from build123d import *

# Parameters (mm, degrees)
PAD006_DEPTH = 4.5
PAD007_DEPTH = 7


with BuildPart() as part:
    # Sketch015 → Revolution (revolve)
    with BuildSketch(Plane.YZ):
        Polygon((0, 4), (8, 4), (8, 0), (6, 0), (6, -6), (8, -6), (8, -12.5), (11.15, -12.5), (11.15, -39), (3.5, -39), (3.5, -62), (4.5, -62), (4.5, -65), (1.9004150762, -65), (0.5, -67), (0, -67), align=None)
    revolve(axis=Axis((0, 0, 0), (0, 0, 1)))

    # Sketch016 → Pad006 (new body)
    with BuildSketch(Plane.XZ):
        Polygon((-3.5, -62), (-15.5, -62), (-15.5, -42), (4.5, -42), (4.5, -62), (3.5, -62), align=None)
    extrude(amount=PAD006_DEPTH)

    # Sketch016 → Pad007 (join)
    with BuildSketch(Plane.XZ):
        Polygon((-3.5, -62), (-15.5, -62), (-15.5, -42), (4.5, -42), (4.5, -62), (3.5, -62), align=None)
    extrude(amount=-PAD007_DEPTH)


solid = part.part
Work out the finished part from the listing and answer in its coordinate system (mm). A direction names the side the tool comes from. Round coordinates to 2 decimals unless told otherwise and drop trailing zeros. Loops run counter-clockwise (first coordinate to the right, second up) from the corner with the lowest first, then second, coordinate; pieces in that order, holes last. Notation, with made-up numbers: (55, 14.25) - (68, 14.25) arc R11 ccw to (68, 22.25) - close; hole circle Ø1 at (-5.75, -34). An arc over 180 degrees is marked (long way). Use one line per item in the form item = value. Start each with the question number.
(1) Flat-ended cylindrical pins translate along their axes: P1, Ø8, axis at x = -12.5, y = -6.5, coming from the -Z side; P2, Ø6, axis at y = 6.5, z = -39.5, coming from the +X side; P3, Ø10, axis at x = -7.5, z = -57, coming from the +Y side; P4, Ø1, axis at y = -6.5, z = -44, coming from the +X side. Find the tip coordinate at first contact, or state that the pin passes through.
(2) Find section B-B on z = -16. Determine the outline of the cut face in (x, y).
(3) Find section C-C on z = -50. Determine the outline of the cut face in (x, y), and give its area (3 significant figures).
(4) Which of the six approach directions +Z, -Z, +X, -X, +Y, -Y give full straight-line access (tool end or side, diameter ignored) to faces 1 (the face through (-8, 3, -12.5)), 2 (the face through (4, -4, -62)), 3 (the face through (-6, -2, 0))?
(5) Consider line 1 (Z direction, x = -9, y = -2); line 2 (Z direction, x = 1, y = -4); line 3 (Z direction, x = 3.5, y = -8). Determine where each line is inside the solid, lowest interval first.
(6) Find section A-A on z = -40.5. Determine the outline of the cut face in (x, y).
Answer list:
q1.P1 = -62
q1.P2 = 10.57
q1.P3 = 7
q1.P4 = through
q2.outline = circle Ø22.3 at (0, 0)
q3.outline = (-15.5, -4.5) - (4.5, -4.5) - (4.5, 7) - (-15.5, 7) - close
q3.area = 230 mm^2
q4.face_1 = +Z
q4.face_2 = -Z, +X, -Y
q4.face_3 = none
q5.line_1 = -62 to -42, -39 to -12.5
q5.line_2 = -65 to -42, -39 to 4
q5.line_3 = -39 to -12.5
q6.outline = circle Ø7 at (0, 0)
